Autodesk Inventor part; units mm, degrees
ref_plane "YZ Plane" through (0, 0, 0) normal (1, 0, 0) x (0, 1, 0)
ref_plane "XZ Plane" through (0, 0, 0) normal (0, 1, 0) x (-1, 0, 0)
ref_plane "XY Plane" through (0, 0, 0) normal (0, 0, 1) x (1, 0, 0)
sketch "Sketch1" plane through (0, 0, 0) normal (0, 0, 1) x (1, 0, 0)
  circle A0 centre (0, 0) radius 37.5
  line L0 (-30, 22.5) -> (-30, -22.5)
  line L1 (30, 22.5) -> (30, -22.5)
  dimension "d0" = 75
  dimension "d20" = 45
extrude "Extrusion1" add sketch "Sketch1" along normal blind 1.5875 contours L1 A0 L0
sketch "Sketch2" plane through (0, 0, 1.5875) normal (0, 0, 1) x (1, 0, 0)
  circle A0 centre (-14, -14) radius 1.75
  line L0 (30, -22.5) -> (30, 22.5)
  line L1 (-30, 22.5) -> (-30, -22.5)
  point P0 (0, 0)
  point P1 (22, -14)
  point P2 (14, 14)
  point P3 (-22, 14)
  point P4 (0, -25)
  point P5 (0, 30)
  dimension "d11" = 8
  dimension "d15" = 16
  dimension "d21" = 16
  dimension "d24" = 8
  dimension "d26" = 28
  dimension "d27" = 28
  dimension "d28" = 14
  dimension "d29" = 14
  dimension "d30" = 25
  dimension "d31" = 30
hole "Hole1" at (22, -14, 1.5875) at (14, 14, 1.5875) at (-14, -14, 1.5875) at (-22, 14, 1.5875) at (0, -25, 1.5875) at (0, 30, 1.5875) direction (0, 0, -1) diameter 3.5 end through all
equation "\"d15\" = d21"
properties part number "PCB_PLACEHOLDER"
Build history of the part. All positions in model axes, mm. Give positions to 0.01 mm unless a question says otherwise; leave off trailing zeros. Order: outer loops, then holes, each group sorted by start corner. A loop starts at its lowest first (then second) coordinate and runs counter-clockwise, first axis right, second up. Notation, with made-up numbers: M -20.5,52 L 17.5,52 A10 ccw 17.5,69 Z; hole C 5.25,48.5 d4. An arc over 180 degrees is marked long. Put each result on its own line as item: value.
Item 1: Flat gauge pin, fed straight in: pin 1 Ø5.5 at (x, y) = (-22, 14) entering from -Z. Where does the tip first touch, or does it go through?
From the geometry:
pin 1: stops at z = 0
Item 2: Two-plate mould, pull along Y, no slides. Class faces 1 (the cylindrical face through (-23.735, 14.228, 0.783)), 2 (the cylindrical face through (-0.08, -23.25, 0.78)), 3 (the flat face through (30, 0, 1)), 4 (the cylindrical face through (0.487, -37.497, 0.783)): +Y half, -Y half, draft (parallel to the pull), parting line (faces both ways), or undercut.
From the geometry:
face 1: undercut
face 2: undercut
face 3: draft
face 4: -Y half
Item 3: Slice it at D-D, the plane y = -25. Write the cut outline in (x, z), plus the area to 3 significant figures.
From the geometry:
outline: M -27.95,0 L -1.75,0 L -1.75,1.59 L -27.95,1.59 Z; M 1.75,0 L 27.95,0 L 27.95,1.59 L 1.75,1.59 Z
area: 83.2 mm2
Item 4: Slice it at C-C, the plane z = 1.3. Write the cut outline in (x, y).
From the geometry:
outline: M -30,-22.5 A37.5 ccw 30,-22.5 L 30,22.5 A37.5 ccw -30,22.5 Z; hole C -22,14 d3.5; hole C -14,-14 d3.5; hole C 0,-25 d3.5; hole C 0,30 d3.5; hole C 14,14 d3.5; hole C 22,-14 d3.5
Item 5: Probe line 1 (X direction, y = 14, z = 1); line 2 (X direction, y = -14, z = 0.7); line 3 (X direction, y = 31.5, z = 1.3). List the from-to ranges inside material, lowest first. Write a range as [from, to].
From the geometry:
line 1: x = [-30, -23.75], [-20.25, 12.25], [15.75, 30]
line 2: x = [-30, -15.75], [-12.25, 20.25], [23.75, 30]
line 3: x = [-20.35, -0.9], [0.9, 20.35]
Item 6: Slice it at B-B, the plane x = 14. Write the cut outline in (y, z), plus the area to 3 significant figures.
From the geometry:
outline: M -34.79,0 L 12.25,0 L 12.25,1.59 L -34.79,1.59 Z; M 15.75,0 L 34.79,0 L 34.79,1.59 L 15.75,1.59 Z
area: 105 mm2
Item 7: Slice it at A-A, the plane y = -14. Write the cut outline in (x, z).
From the geometry:
outline: M -30,0 L -15.75,0 L -15.75,1.59 L -30,1.59 Z; M -12.25,0 L 20.25,0 L 20.25,1.59 L -12.25,1.59 Z; M 23.75,0 L 30,0 L 30,1.59 L 23.75,1.59 Z
